```python
from build123d import *
from OCP.BRepFilletAPI import BRepFilletAPI_MakeChamfer

# Parameters (mm, degrees)
SKETCH1_W               = 72
SKETCH1_H               = 85
SKETCH1_R               = 2
BOSS_EXTRUDE1_DEPTH     = 5
SKETCH2_W               = 5
SKETCH2_H               = 15
SKETCH2_W_2             = 62
SKETCH2_H_2             = 2
SKETCH2_H_3             = 35
BOSS_EXTRUDE2_DEPTH     = 40
CUT_EXTRUDE1_DEPTH      = 5
CUT_EXTRUDE_THIN1_DEPTH = 5
FILLET1_R               = 10
CHAMFER1_SIZE           = 37
CHAMFER1_SIZE2          = 21.36195996
CHAMFER2_SIZE           = 30
CHAMFER2_SIZE2          = 8.038475773
FILLET2_R               = 2
FILLET4_R               = 5


with BuildPart() as part:
    # Sketch1 → Boss-Extrude1 (new body)
    with BuildSketch(Plane(origin=(0, 0, 0), x_dir=(1, 0, 0), z_dir=(0, 1, 0))):
        with Locations((26, 32.5)):
            Rectangle(SKETCH1_W, SKETCH1_H)
        with Locations(Location((0, 65, 0), (0, 0, 270))):
            Circle(SKETCH1_R, mode=Mode.SUBTRACT)
        with Locations(Location((52, 65, 0), (0, 0, 270))):
            Circle(SKETCH1_R, mode=Mode.SUBTRACT)
        with Locations(Location((52, 0, 0), (0, 0, 270))):
            Circle(SKETCH1_R, mode=Mode.SUBTRACT)
    extrude(amount=BOSS_EXTRUDE1_DEPTH)

    # Sketch2 → Boss-Extrude2 (add)
    with BuildSketch(Plane(origin=(0, 5, 0), x_dir=(1, 0, 0), z_dir=(0, 1, 0))):
        with Locations((-2.5, 12.5)):
            Rectangle(SKETCH2_W, SKETCH2_H)
        with Locations((26, 21)):
            Rectangle(SKETCH2_W_2, SKETCH2_H_2)
        with Locations((54.5, 12.5)):
            Rectangle(SKETCH2_W, SKETCH2_H)
        with Locations((54.5, 39.5)):
            Rectangle(SKETCH2_W, SKETCH2_H_3)
        with Locations((-2.5, 39.5)):
            Rectangle(SKETCH2_W, SKETCH2_H_3)
    extrude(amount=BOSS_EXTRUDE2_DEPTH)

    # Sketch3 → Cut-Extrude1 (cut)
    with BuildSketch(Plane.XY.offset(-20)):
        Polygon((26, 35), (30.55, 35), (30.55, 29.35), (39, 29.35), (39, 18.75), (35.5, 18.75), (35.5, 13), (16.5, 13), (16.5, 18.75), (13, 18.75), (13, 29.35), (21.45, 29.35), (21.45, 35), align=None)
    extrude(amount=-CUT_EXTRUDE1_DEPTH, mode=Mode.SUBTRACT)

    # Sketch3_3 → Cut-Extrude-Thin1 (cut)
    with BuildSketch(Plane.XY.offset(-20)):
        Polygon((26, 35.75), (31.3, 35.75), (31.3, 30.1), (39.75, 30.1), (39.75, 18), (36.25, 18), (36.25, 12.25), (15.75, 12.25), (15.75, 18), (12.25, 18), (12.25, 30.1), (20.7, 30.1), (20.7, 35.75), align=None)
        Polygon((26, 35), (30.55, 35), (30.55, 29.35), (39, 29.35), (39, 18.75), (35.5, 18.75), (35.5, 13), (16.5, 13), (16.5, 18.75), (13, 18.75), (13, 29.35), (21.45, 29.35), (21.45, 35), align=None, mode=Mode.SUBTRACT)
    extrude(amount=-CUT_EXTRUDE_THIN1_DEPTH, mode=Mode.SUBTRACT)

    # Fillet1
    fillet1_edges = [part.edges().sort_by_distance(p)[0] for p in [
        (0, 25, -20),
        (52, 25, -20),
        (52, 25, -22),
        (0, 25, -22),
    ]]
    fillet(fillet1_edges, radius=FILLET1_R)

    # Chamfer1: one chamfer whose edges measure the first distance from different faces: ONE call of the kernel's chamfer builder (chamfer() names one face for all edges)
    chamfer1_edges_1 = [part.edges().sort_by_distance(p)[0] for p in [
        (-2.5, 45, -57),
    ]]
    chamfer1_side_1 = [part.faces().sort_by_distance(p)[0] for p in [
        (-2.5, 25, -57),
    ]]
    chamfer1_edges_2 = [part.edges().sort_by_distance(p)[0] for p in [
        (54.5, 45, -57),
    ]]
    chamfer1_side_2 = [part.faces().sort_by_distance(p)[0] for p in [
        (54.5, 25, -57),
    ]]
    chamfer1 = BRepFilletAPI_MakeChamfer(part.part.solid().wrapped)
    for e in chamfer1_edges_1:
        chamfer1.Add(CHAMFER1_SIZE, CHAMFER1_SIZE2, e.wrapped, chamfer1_side_1[0].wrapped)  # the first distance lies on this face
    for e in chamfer1_edges_2:
        chamfer1.Add(CHAMFER1_SIZE, CHAMFER1_SIZE2, e.wrapped, chamfer1_side_2[0].wrapped)  # the first distance lies on this face
    add(Compound.cast(chamfer1.Shape()), mode=Mode.REPLACE)

    # Chamfer2: one chamfer whose edges measure the first distance from different faces: ONE call of the kernel's chamfer builder (chamfer() names one face for all edges)
    chamfer2_edges_1 = [part.edges().sort_by_distance(p)[0] for p in [
        (54.5, 45, -5),
    ]]
    chamfer2_side_1 = [part.faces().sort_by_distance(p)[0] for p in [
        (54.5, 25, -5),
    ]]
    chamfer2_edges_2 = [part.edges().sort_by_distance(p)[0] for p in [
        (-2.5, 45, -5),
    ]]
    chamfer2_side_2 = [part.faces().sort_by_distance(p)[0] for p in [
        (-2.5, 25, -5),
    ]]
    chamfer2 = BRepFilletAPI_MakeChamfer(part.part.solid().wrapped)
    for e in chamfer2_edges_1:
        chamfer2.Add(CHAMFER2_SIZE, CHAMFER2_SIZE2, e.wrapped, chamfer2_side_1[0].wrapped)  # the first distance lies on this face
    for e in chamfer2_edges_2:
        chamfer2.Add(CHAMFER2_SIZE, CHAMFER2_SIZE2, e.wrapped, chamfer2_side_2[0].wrapped)  # the first distance lies on this face
    add(Compound.cast(chamfer2.Shape()), mode=Mode.REPLACE)

    # Fillet2
    fillet2_edges = [part.edges().sort_by_distance(p)[0] for p in [
        (0, 5, -44.5),
        (0, 5, -7.5),
        (26, 5, -22),
        (52, 5, -44.5),
        (52, 5, -7.5),
        (26, 5, -20),
        (2.928932188, 5, -17.071067812),
        (49.071067812, 5, -17.071067812),
        (49.071067812, 5, -24.928932188),
        (2.928932188, 5, -24.928932188),
        (57, 5, -31),
        (54.5, 5, -57),
        (-5, 5, -31),
        (-2.5, 5, -5),
        (-2.5, 5, -57),
        (54.5, 5, -5),
    ]]
    fillet(fillet2_edges, radius=FILLET2_R)

    # Fillet4
    fillet4_edges = [part.edges().sort_by_distance(p)[0] for p in [
        (-2.263603284, 45, -13.038475773),
        (54.263603284, 45, -13.038475773),
        (54.5, 45, -35.63804004),
        (-2.5, 45, -35.63804004),
        (62, 2.5, -75),
        (62, 2.5, 10),
        (-10, 2.5, -75),
        (-10, 2.5, 10),
    ]]
    fillet(fillet4_edges, radius=FILLET4_R)


solid = part.part
```
The model under review builds one solid part; all positions refer to its coordinate system, in mm. A direction names the side the tool comes from. Round coordinates to 2 decimals unless told otherwise and drop trailing zeros. Write each loop counter-clockwise with the first axis right and the second up, starting at its lowest first coordinate (ties: lowest second). Pieces come first, ordered by that corner, then holes. Notation, with made-up numbers: (87, 69) - (115, 69) arc R25 ccw to (115, 97) - close; hole circle Ø1 at (63.5, 61). An arc over 180 degrees is marked (long way). Use one line per item in the form item = value.
Q1. Insertion check: pin 1 Ø3 at (y, z) = (10, -57) entering from -X; pin 2 Ø2 at (x, y) = (38.5, 27.5) entering from +Z; pin 3 Ø1.6 at (y, z) = (22.5, -21) entering from +X; pin 4 Ø16 at (x, y) = (32.5, 31.5) entering from +Z. Each pin has a flat end and moves straight along its axis. Give the tip position at first contact, or say it passes through.
Answer key:
pin_1 = -5
pin_2 = through
pin_3 = 57
pin_4 = -20
Q2. Consider section B-B (z = 0). State the section outline as (x, y) points.
Answer key:
outline = (-10, 0) - (50, 0) - (50, 5) - (-10, 5) - close; (54, 0) - (62, 0) - (62, 5) - (54, 5) - close
Q3. Tool access review of faces 4 (the flat face through (0, 17, -8)), 5 (the flat face through (14, 18, -21)), 6 (the cylindrical face through (49.15, 26.27, -25.01)): name each direction out of +Z, -Z, +X, -X, +Y, -Y from which nothing blocks a thin tool from reaching the whole face with its end or side.
Answer key:
face_4 = +Z, +Y
face_5 = +Z, -Z
face_6 = -Z, +Y
Q4. Consider section C-C (z = -9). State the section outline as (x, y) points, and give its area (3 significant figures).
Answer key:
outline = (-10, 0) - (62, 0) - (62, 5) - (59, 5) arc R2 cw to (57, 7) - (57, 29.93) - (52, 29.93) - (52, 7) arc R2 cw to (50, 5) - (2, 5) arc R2 cw to (0, 7) - (0, 29.93) - (-5, 29.93) - (-5, 7) arc R2 cw to (-7, 5) - (-10, 5) - close
area = 613 mm2
Q5. Consider section A-A (z = -65). State the section outline as (x, y) points.
Answer key:
outline = (-10, 0) - (-2, 0) - (-2, 5) - (-10, 5) - close; (2, 0) - (50, 0) - (50, 5) - (2, 5) - close; (54, 0) - (62, 0) - (62, 5) - (54, 5) - close
Q6. For line 1 (X direction, y = 25, z = -37); line 2 (Y direction, x = 44.5, z = -10); line 3 (Z direction, x = 23.5, y = 42), list the stretches that pass through material, from the lowest coordinate up. Write a range as [from, to].
Answer key:
line_1 = [-5, 0], [52, 57]
line_2 = [0, 5]
line_3 = [-22, -20]
Q7. Draft analysis for pull direction Z (two halves, no side actions). For faces 1 (the cylindrical face through (-0.766, 2.465, -63.153)), 2 (the flat face through (25, 5, -33)), 3 (the flat face through (26, 2, -75)), state which applies: +Z half, -Z half, draft (parallel to the pull), parting line (faces both ways), or undercut.
Answer key:
face_1 = undercut
face_2 = draft
face_3 = -Z half
